Work out the finished part from the listing and answer in its coordinate system (mm). Face numbers are marked on the shaded views. A direction names the side the tool comes from. Coordinates: 2 decimals unless noted, no trailing zeros. Order: outer loops, then holes, each group sorted by start corner. A loop starts at its lowest first (then second) coordinate and runs counter-clockwise, first axis right, second up. Notation, with made-up numbers: M -31,5 L -13,5 A20 cw -13,21 Z; hole C 76.5,-14 d1. An arc over 180 degrees is marked long. Use a Markdown table: item, result.
from build123d import *

# Parameters (mm, degrees)
SKETCH2_W           = 23
SKETCH2_H           = 12
BOSS_EXTRUDE1_DEPTH = 23
BOSS_EXTRUDE2_START = -4.4
BOSS_EXTRUDE2_DEPTH = 2.4
SKETCH4_R           = 6
SKETCH4_R_2         = 2.5
BOSS_EXTRUDE3_DEPTH = 4.3
BOSS_EXTRUDE4_DEPTH = 3
SKETCH6_W           = 3
SKETCH6_H           = 1
BOSS_EXTRUDE5_DEPTH = 3


with BuildPart() as part:
    # Sketch2 → Boss-Extrude1 (new body)
    with BuildSketch(Plane(origin=(0, 0, 0), x_dir=(1, 0, 0), z_dir=(0, 1, 0))):
        Rectangle(SKETCH2_W, SKETCH2_H)
    extrude(amount=-BOSS_EXTRUDE1_DEPTH)

    # Sketch3 → Boss-Extrude2 (add)
    with BuildSketch(Plane(origin=(0, 0, 0), x_dir=(1, 0, 0), z_dir=(0, 1, 0)).offset(BOSS_EXTRUDE2_START)):
        with BuildLine():
            Line((-16.2, -0.5), (-16.2, -6))
            Line((-16.2, -6), (-11.5, -6))
            Line((-11.5, -6), (-11.5, 6))
            Line((-11.5, 6), (-16.2, 6))
            Line((-16.2, 6), (-16.2, 0.5))
            Line((-16.2, 0.5), (-15.584293743, 0.5))
            ThreePointArc((-15.584293743, 0.5), (-14.459449294, 0.965925826), (-13.718268339, 0))
            ThreePointArc((-13.718268339, 0), (-14.459449294, -0.965925826), (-15.584293743, -0.5))
            Line((-15.584293743, -0.5), (-16.2, -0.5))
        make_face()
        with BuildLine():
            Line((11.5, 6), (11.5, -6))
            Line((11.5, -6), (16.2, -6))
            Line((16.2, -6), (16.2, -0.5))
            Line((16.2, -0.5), (14.894380034, -0.5))
            ThreePointArc((14.894380034, -0.5), (13.02835463, 0), (14.894380034, 0.5))
            Line((14.894380034, 0.5), (16.2, 0.5))
            Line((16.2, 0.5), (16.2, 6))
            Line((16.2, 6), (11.5, 6))
        make_face()
    extrude(amount=-BOSS_EXTRUDE2_DEPTH)

    # Sketch4 → Boss-Extrude3 (add)
    with BuildSketch(Plane(origin=(0, 0, 0), x_dir=(1, 0, 0), z_dir=(0, 1, 0))):
        with Locations((-5.5, 0)):
            Circle(SKETCH4_R)
        with Locations((0.8, 0)):
            Circle(SKETCH4_R_2)
    extrude(amount=BOSS_EXTRUDE3_DEPTH)

    # Sketch5 → Boss-Extrude4 (add)
    with BuildSketch(Plane(origin=(0, 4.3, 0), x_dir=(1, 0, 0), z_dir=(0, 1, 0))):
        Polygon((-3.255005568, -0.15), (-3.437184296, 0), (-3.255005568, 0.15), (-3.455589794, 0.274946425), (-3.295142762, 0.44844683), (-3.51047784, 0.544986424), (-3.374587739, 0.738324266), (-3.600868956, 0.805301127), (-3.491960749, 1.015026288), (-3.725150111, 1.051245213), (-3.645167266, 1.273615142), (-3.881103504, 1.278429803), (-3.831473318, 1.509476304), (-4.065946143, 1.482800783), (-4.047554268, 1.718400825), (-4.276379508, 1.660711148), (-4.289554146, 1.896660443), (-4.508648409, 1.808986083), (-4.553154459, 2.04107411), (-4.758608002, 1.924979619), (-4.833651254, 2.149064761), (-5.021797754, 2.006621847), (-5.126039057, 2.218705301), (-5.293521035, 2.052455862), (-5.425100203, 2.248752992), (-5.568928939, 2.061663752), (-5.725497937, 2.238671633), (-5.843106805, 2.034081205), (-6.021871655, 2.188641125), (-6.111161921, 1.97020043), (-6.308932561, 2.099554265), (-6.368310838, 1.871161381), (-6.581558046, 1.973000809), (-6.609964728, 1.738731414), (-6.834883102, 1.811239107), (-6.831811271, 1.575273743), (-7.064387138, 1.6171558), (-7.02989161, 1.383705275), (-7.265974648, 1.39421431), (-7.200670997, 1.167444554), (-7.436048299, 1.146393032), (-7.34110187, 0.930350756), (-7.571573122, 0.878114343), (-7.448678237, 0.676654828), (-7.670130674, 0.594165683), (-7.521480394, 0.410883978), (-7.729962192, 0.299614123), (-7.558209186, 0.137780894), (-7.749999982, -0.000284059), (-7.558209186, -0.137780894), (-7.729886469, -0.300177172), (-7.521480394, -0.410883978), (-7.669980579, -0.594713616), (-7.448678237, -0.676654828), (-7.571351335, -0.878637381), (-7.34110187, -0.930350756), (-7.435758777, -1.146881842), (-7.200670997, -1.167444554), (-7.265622557, -1.394660168), (-7.02989161, -1.383705275), (-7.063978761, -1.617550752), (-6.831811271, -1.575273743), (-6.834425728, -1.811576103), (-6.609964728, -1.738731414), (-6.581059835, -1.973273836), (-6.368310838, -1.871161381), (-6.308402404, -2.099758451), (-6.111161921, -1.97020043), (-6.021319013, -2.188772827), (-5.843106805, -2.034081205), (-5.724932672, -2.238728499), (-5.568928939, -2.061663752), (-5.424532402, -2.248734009), (-5.293521035, -2.052455862), (-5.125478853, -2.218610806), (-5.021797754, -2.006621847), (-4.833108643, -2.148896442), (-4.758608002, -1.924979619), (-4.552639125, -2.040834969), (-4.508648409, -1.808986083), (-4.289075284, -1.896354748), (-4.276379508, -1.660711148), (-4.047120423, -1.718034032), (-4.065946143, -1.482800783), (-3.831092233, -1.509054958), (-3.881103504, -1.278429803), (-3.644845742, -1.273146762), (-3.725150111, -1.051245213), (-3.491704522, -1.014519232), (-3.600868956, -0.805301127), (-3.374401382, -0.737787582), (-3.51047784, -0.544986424), (-3.295029601, -0.447890096), (-3.455589794, -0.274946425), align=None)
    extrude(amount=BOSS_EXTRUDE4_DEPTH)

    # Sketch6 → Boss-Extrude5 (add)
    with BuildSketch(Plane.ZY.offset(11.5)):
        with Locations((0, -17.5)):
            Rectangle(SKETCH6_W, SKETCH6_H)
    extrude(amount=BOSS_EXTRUDE5_DEPTH)


solid = part.part
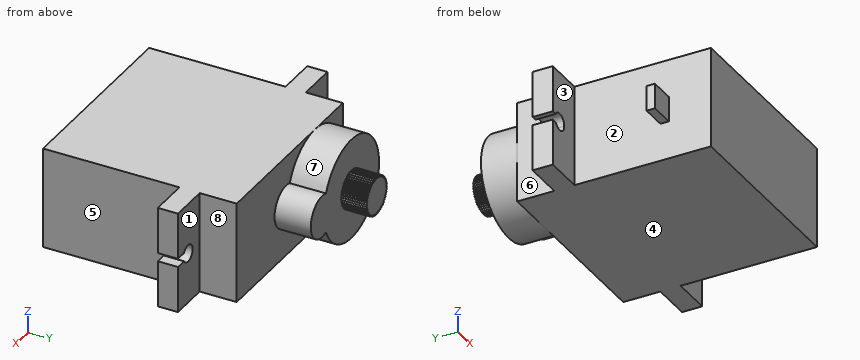
1. Section C-C on z = -4 is taken. Determine the outline of the cut face in (x, y).
Answers below:
| item | result |
|---|---|
| outline | M -16.2,-6.8 L -11.5,-6.8 L -11.5,-23 L 11.5,-23 L 11.5,-6.8 L 16.2,-6.8 L 16.2,-4.4 L 11.5,-4.4 L 11.5,0 L -1.03,0 L -1.03,4.3 L -9.97,4.3 L -9.97,0 L -11.5,0 L -11.5,-4.4 L -16.2,-4.4 Z |
2. Find the intervals of material crossed by probe 1 along X at (y, z) = (-5.8, 0); probe 2 along X at (y, z) = (-20, -5); probe 3 along Y at (x, z) = (-3, 3.25), in increasing order.
Answers below:
| item | result |
|---|---|
| probe 1 | -13.72 to 13.03 |
| probe 2 | -11.5 to 11.5 |
| probe 3 | -23 to 4.3 |
3. For a pull along Y with two mould halves and no side action, classify the marked faces 1, 2, 3 and 4 as +Y half, -Y half, draft (parallel to the pull), parting line (faces both ways), or undercut.
Answers below:
| item | result |
|---|---|
| face 1 | +Y half |
| face 2 | undercut |
| face 3 | undercut |
| face 4 | draft |
4. Flat-ended cylindrical pins translate along their axes: P1, Ø1, axis at x = 1, z = -4, coming from the +Y side; P2, Ø3, axis at x = -7.5, z = 2.5, coming from the +Y side; P3, Ø6.5, axis at x = -10, z = -3.5, coming from the +Y side; P4, Ø0.5, axis at x = -13.5, y = -17.5, coming from the -Z side. Find the tip coordinate at first contact, or state that the pin passes through.
Answers below:
| item | result |
|---|---|
| P1 | y = 0 |
| P2 | y = 7.3 |
| P3 | y = 4.3 |
| P4 | z = -1.5 |
5. Section D-D on y = -11.5 is taken. Determine the outline of the cut face in (x, z), then the cut area to 3 significant figures.
Answers below:
| item | result |
|---|---|
| outline | M -11.5,-6 L 11.5,-6 L 11.5,6 L -11.5,6 Z |
| area | 276 mm² |
6. For the marked faces 5, 6, 7 and 8, determine the directions among +Z, -Z, +X, -X, +Y, -Y from which every point of the face is accessible in a straight line to the end or side of a thin tool.
Answers below:
| item | result |
|---|---|
| face 5 | +Z, -Z, +X, -Y |
| face 6 | +Z, -Z, -X, +Y |
| face 7 | +Y |
| face 8 | +Z, -Z, +X, +Y |
7. Section B-B on x = 0.8 is taken. Determine the outline of the cut face in (y, z), then the cut area to 4 significant figures.
Answers below:
| item | result |
|---|---|
| outline | M -23,-6 L 0,-6 L 0,-2.5 L 4.3,-2.5 L 4.3,2.5 L 0,2.5 L 0,6 L -23,6 Z |
| area | 297.5 mm² |
8. Section A-A on x = 14.5 is taken. Determine the outline of the cut face in (y, z).
Answers below:
| item | result |
|---|---|
| outline | M -6.8,-6 L -4.4,-6 L -4.4,-0.88 L -6.8,-0.88 Z; M -6.8,0.88 L -4.4,0.88 L -4.4,6 L -6.8,6 Z |
